```python
from build123d import *

# Parameters (mm, degrees)
F1_DEPTH = 5.08
F2_R     = 6.35
F3_DEPTH = 5.081


# Not quite as in the source:
# - a feature names something its author has since deleted; it is built from what else it names


with BuildPart() as f1:
    # F0 (on Front) → F1 (new body)
    with BuildSketch(Plane.XZ):
        with BuildLine():
            Line((137.8481502717, 12.7), (79.9225977639, 113.03))
            ThreePointArc((79.9225977639, 113.03), (70.6255525078, 122.3270452561), (57.9255525078, 125.73))
            Line((57.9255525078, 125.73), (-57.9255525078, 125.73))
            ThreePointArc((-57.9255525078, 125.73), (-70.6255525078, 122.3270452561), (-79.9225977639, 113.03))
            Line((-79.9225977639, 113.03), (-137.8481502717, 12.7))
            ThreePointArc((-137.8481502717, 12.7), (-141.2511050156, 0), (-137.8481502717, -12.7))
            Line((-137.8481502717, -12.7), (-79.9225977639, -113.03))
            ThreePointArc((-79.9225977639, -113.03), (-70.6255525078, -122.3270452561), (-57.9255525078, -125.73))
            Line((-57.9255525078, -125.73), (57.9255525078, -125.73))
            ThreePointArc((57.9255525078, -125.73), (70.6255525078, -122.3270452561), (79.9225977639, -113.03))
            Line((79.9225977639, -113.03), (137.8481502717, -12.7))
            ThreePointArc((137.8481502717, -12.7), (141.2511050156, 0), (137.8481502717, 12.7))
        make_face()
    extrude(amount=F1_DEPTH)

    # F2 (on face) → F3 (cut, through all)
    with BuildSketch(Plane.XZ.offset(5.08)):
        with Locations((0, 109.855)):
            Circle(F2_R)
        with Locations((-95.1372207327, -54.9275)):
            Circle(F2_R)
        with Locations((95.1372207327, -54.9275)):
            Circle(F2_R)
    extrude(amount=-F3_DEPTH, mode=Mode.SUBTRACT)


solid = f1.part
```
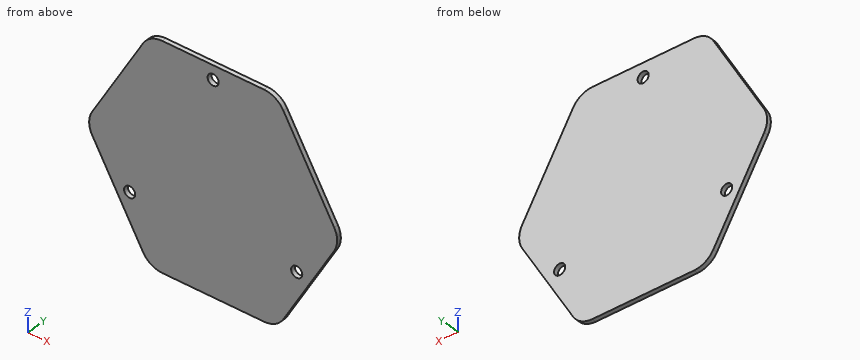
Model file for the job. Use its own axes, mm. Give positions to 0.01 mm unless a question says otherwise; leave off trailing zeros. Loops run counter-clockwise (first coordinate to the right, second up) from the corner with the lowest first, then second, coordinate; pieces in that order, holes last. Notation, with made-up numbers: M -30,74.5 L 14,74.5 A20 ccw 14,88.5 Z; hole C 65,28 d10. An arc over 180 degrees is marked long. Use one line per item in the form item = value.
Item 1: Drill centre lines: L1, parallel to X at y = -0.15, z = 112; L2, parallel to X at y = -4.1, z = -56; L3, parallel to Z at x = -92.5, y = -4.25. Where is each one in solid material? Low to high.
Filled in:
L1 = -80.52 to -5.98, 5.98 to 80.52
L2 = -112.85 to -101.4, -88.88 to 88.88, 101.4 to 112.85
L3 = -91.25 to -60.7, -49.15 to 91.25
Item 2: Slice it at B-B on y = -3.65. Give the number of separate pieces and of enclosed holes in the cut face, and give its area (3 significant figures).
Filled in:
separate_pieces = 1
enclosed_holes = 3
area = 54,200 mm^2
Item 3: Flat gauge pins, fed straight in: pin 1 Ø1 at (x, y) = (-80, -4) entering from -Z; pin 2 Ø8 at (x, z) = (-89.5, -35.5) entering from +Y; pin 3 Ø1 at (x, y) = (-78.5, -3.5) entering from -Z. Where does each tip first touch, or does it go through?
Filled in:
pin_1 = -113.74
pin_2 = 0
pin_3 = -115.89
Item 4: Slice it at C-C on x = -95. List the corners of the cut face in (y, z), and give its area (3 significant figures).
Filled in:
outline = M -5.08,-86.92 L 0,-86.92 L 0,-61.28 L -5.08,-61.28 Z; M -5.08,-48.58 L 0,-48.58 L 0,86.92 L -5.08,86.92 Z
area = 819 mm^2
Item 5: Slice it at D-D on z = 90.5. List the corners of the cut face in (x, y), and give its area (3 significant figures).
Filled in:
outline = M -92.93,-5.08 L 92.93,-5.08 L 92.93,0 L -92.93,0 Z
area = 944 mm^2
Item 6: Slice it at A-A on x = 0. List the corners of the cut face in (y, z) (3 decimals).
Filled in:
outline = M -5.08,-125.73 L 0,-125.73 L 0,103.505 L -5.08,103.505 Z; M -5.08,116.205 L 0,116.205 L 0,125.73 L -5.08,125.73 Z
